Verification items for this drawing (mm, ordinates from the low corner). A direction names the side the tool comes from. Round coordinates to 2 decimals unless told otherwise and drop trailing zeros. Write each loop counter-clockwise with the first axis right and the second up, starting at its lowest first coordinate (ties: lowest second). Pieces come first, ordered by that corner, then holes. Notation, with made-up numbers: (76, 6.5) -> (107, 6.5) arc R14 cw to (107, 23.5) -> close; hole circle Ø8 at (-29.5, 26.5). An arc over 180 degrees is marked (long way). Return JSON: item names as keys, results as strings. Group by question number.
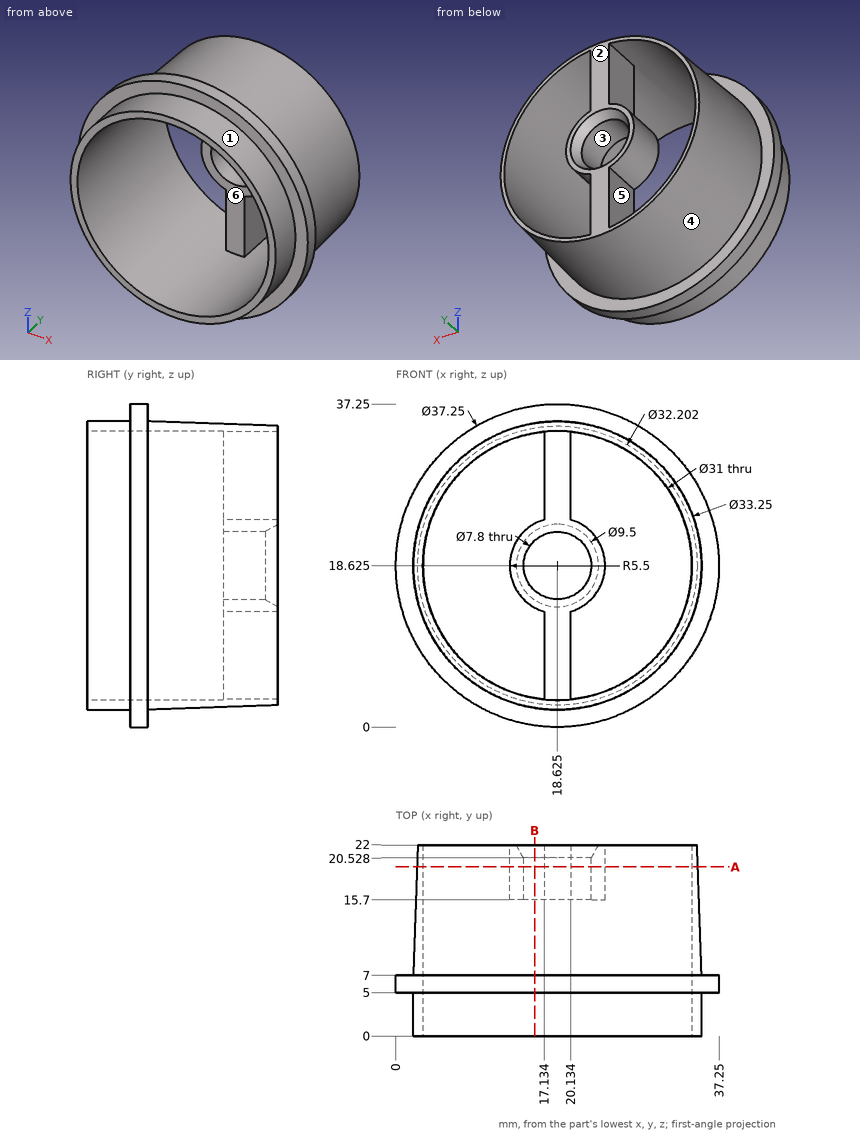
1) Material ranges on probe 1 along X at (y, z) = (16.5, 17.5) (1 decimal); probe 2 along Z at (x, y) = (32, 16) (1 decimal); probe 3 along X at (y, z) = (19.75, 6) (1 decimal), recorded low to high. Write a range as [from, to].
2) Sectioned sample at A-A on y = 19.5. Enter the section's corners in (x, z) (1 decimal), and give its area (3 significant figures).
3) Go/stop test with flat-tipped pins: P1, Ø2, axis at x = 24.5, y = 11, coming from the +Z side (1 decimal); P2, Ø5, axis at y = 20.5, z = 26.5, coming from the +X side; P3, Ø1.9, axis at y = 20, z = 9.5, coming from the +X side. Record where each tip stops, or that it passes through.
4) Mould release check, pull along X, two halves, no side actions. Record for the marked faces 1, 2 and 3: +X half, -X half, draft (parallel to the pull), parting line (faces both ways), or undercut.
5) Sectioned sample at B-B on x = 16. State how many separate pieces and enclosed holes the cut face has.
6) Tool access check on the marked faces 4, 5 and 6. Record the directions out of +Z, -Z, +X, -X, +Y, -Y that give a thin tool (end or side, any length) a straight path to the whole face; none if there is none.
Evaluation:
{
 "1": {"probe 1": "x = [2.4, 3.2], [13.2, 14.9], [22.4, 24], [34.1, 34.9]", "probe 2": "z = [9.3, 10.8], [26.5, 28]", "probe 3": "x = [8.5, 9.6], [17.1, 20.1], [27.6, 28.7]"},
 "2": {"outline": "circle Ø32.4 at (18.6, 18.6); hole circle Ø7.8 at (18.6, 18.6); hole (17.1, 3.2) -> (17.1, 13.3) arc R5.5 cw to (17.1, 23.9) -> (17.1, 34.1) arc R15.5 ccw to start; hole (20.1, 3.2) arc R15.5 ccw to (20.1, 34.1) -> (20.1, 23.9) arc R5.5 cw to (20.1, 13.3) -> close", "area": "176 mm2"},
 "3": {"P1": "stops at z = 34.4", "P2": "stops at x = 33.86", "P3": "stops at x = 32.58"},
 "4": {"face 1": "parting line", "face 2": "draft", "face 3": "undercut"},
 "5": {"separate pieces": "4", "enclosed holes": "0"},
 "6": {"face 4": "+Y", "face 5": "+Y, -Y", "face 6": "-Y"}
}
